from build123d import *

# Parameters (mm, degrees)
SKETCH1_R           = 14.0975
SKETCH1_R_2         = 12.7
BOSS_EXTRUDE1_DEPTH = 152.5
SKETCH2_W           = 29.43875972
SKETCH2_H           = 15.555523124
CUT_EXTRUDE1_DEPTH  = 27.5
SKETCH3_W           = 13
SKETCH3_H           = 5.253170184
CUT_EXTRUDE2_DEPTH  = 6.5
FILLET1_R           = 2.38
SKETCH4_W           = 35.595029472
SKETCH4_H           = 37.761683439
CUT_EXTRUDE3_DEPTH  = 2.25


with BuildPart() as part:
    # Sketch1 → Boss-Extrude1 (new body)
    with BuildSketch(Plane(origin=(0, 0, 0), x_dir=(1, 0, 0), z_dir=(0, 1, 0))):
        with Locations(Location((0, 0, 0), (0, 0, 270))):
            Circle(SKETCH1_R)
        with Locations(Location((0, 0, 0), (0, 0, 270))):
            Circle(SKETCH1_R_2, mode=Mode.SUBTRACT)
    extrude(amount=BOSS_EXTRUDE1_DEPTH)

    # Sketch2 → Cut-Extrude1 (cut)
    with BuildSketch(Plane(origin=(0, 152.5, 0), x_dir=(1, 0, 0), z_dir=(0, 1, 0))):
        with Locations((0.62187986, 7.777761562)):
            Rectangle(SKETCH2_W, SKETCH2_H)
    extrude(amount=-CUT_EXTRUDE1_DEPTH, mode=Mode.SUBTRACT)

    # Sketch3 → Cut-Extrude2 (cut)
    with BuildSketch(Plane(origin=(0, 152.5, 0), x_dir=(1, 0, 0), z_dir=(0, 1, 0))):
        with Locations((0, -11.873414908)):
            Rectangle(SKETCH3_W, SKETCH3_H)
    extrude(amount=-CUT_EXTRUDE2_DEPTH, mode=Mode.SUBTRACT)

    # Fillet1
    fillet1_edges = [part.edges().sort_by_distance(p)[0] for p in [
        (6.5, 146, 11.71006097),
        (-6.5, 146, 11.71006097),
    ]]
    fillet(fillet1_edges, radius=FILLET1_R)

    # Sketch4 → Cut-Extrude3 (cut)
    with BuildSketch(Plane.XZ):
        with Locations((0.67063099, 0.361108995)):
            Rectangle(SKETCH4_W, SKETCH4_H)
    extrude(amount=-CUT_EXTRUDE3_DEPTH, mode=Mode.SUBTRACT)


solid = part.part
Could you check a few things on this model? Use its own coordinates, in mm. A direction names the side the tool comes from. Give positions to 0.01 mm unless a question says otherwise; leave off trailing zeros. Write each loop counter-clockwise with the first axis right and the second up, starting at its lowest first coordinate (ties: lowest second). Pieces come first, ordered by that corner, then holes. Notation, with made-up numbers: (-0.5, 33.5) -> (21.5, 33.5) arc R27 cw to (21.5, 58.5) -> close; hole circle Ø4 at (75.25, -18). An arc over 180 degrees is marked (long way). Answer as CSV lines item,"result". Start each with the question number.
(1) If we section it at C-C, the plane y = 51.5: Write out the boundary of the cut face in (x, z) (1 decimal), and give its area (3 significant figures).
(2) If we mould it in two halves opening along X, with no side actions, what happens to faces 1 (the face through (4.23, 76.32, 13.45)), 2 (the face through (-5.784, 146.679, 12.178)), 3 (the face through (-11, 152.5, 7))? For each: +X half, -X half, draft (parallel to the pull), parting line (faces both ways), or undercut.
(3) Please list where these lines run through material, in increasing order: line 1 (X direction, y = 64, z = 0); line 2 (Y direction, x = -6.5, z = -11).
(4) I'm going to push flat-ended pins straight in: pin 1 Ø1 at (x, z) = (0, 13) entering from +Y; pin 2 Ø7 at (x, z) = (0.5, -7) entering from +Y; pin 3 Ø4 at (y, z) = (124.5, 4) entering from +X; pin 4 Ø6 at (x, y) = (-5.5, 125.5) entering from +Z. Where does each tip first touch, or does it pass through?
(5) If we section it at B-B, the plane z = 5.75: Write out the boundary of the cut face in (x, y), and give its area (3 significant figures).
(6) If we section it at A-A, the plane x = 0: Write out the boundary of the cut face in (y, z).
(7) Which directions (+Z, -Z, +X, -X, +Y, -Y) give clear straight access to the entire face, cutting with the end or side of a thin tool? Please do faces 4 (the face through (5.784, 146.679, 12.178)), 5 (the face through (-12, 2.25, 5)), 6 (the face through (-1, 125, -13)).
Answer list:
1,outline,"circle Ø28.2 at (0, 0); hole circle Ø25.4 at (0, 0)"
1,area,"118 mm^2"
2,face 1,"parting line"
2,face 2,"undercut"
2,face 3,"draft"
3,line 1,"-14.1 to -12.7, 12.7 to 14.1"
3,line 2,"2.25 to 125"
4,pin 1,"y = 146"
4,pin 2,"through"
4,pin 3,"x = 13.95"
4,pin 4,"z = 13.87"
5,outline,"(-12.87, 2.25) -> (-11.32, 2.25) -> (-11.32, 152.5) -> (-12.87, 152.5) -> close; (11.32, 2.25) -> (12.87, 2.25) -> (12.87, 152.5) -> (11.32, 152.5) -> close"
5,area,"465 mm^2"
6,outline,"(2.25, -14.1) -> (125, -14.1) -> (125, -12.7) -> (2.25, -12.7) -> close; (2.25, 12.7) -> (146, 12.7) -> (146, 14.1) -> (2.25, 14.1) -> close"
7,face 4,"+Z, -Z, +Y"
7,face 5,"+Z, -Z, +X, -X, -Y"
7,face 6,"-Z, +X, -X, +Y"
